```python
from build123d import *

# Parameters (mm, degrees)
F1_DEPTH = 60.325
F2_DEPTH = 11.1125
F4_DEPTH = 11.1125
F0_W     = 11.1125
F0_H     = 33.3375
F5_DEPTH = 50.8
F6_DEPTH = 25.4
F8_DEPTH = 11.1125


with BuildPart() as f1:
    # F0 (on Top) → F1 (new body)
    with BuildSketch(Plane.XY):
        Polygon((114.3, 0), (0, 0), (0, -11.1125), (11.1125, -11.1125), (63.5, -11.1125), (114.3, -11.1125), align=None)
    extrude(amount=F1_DEPTH)

    # F0 (on Top) → F2 (join)
    with BuildSketch(Plane.XY):
        Polygon((63.5, -11.1125), (11.1125, -11.1125), (11.1125, -44.45), align=None)
    extrude(amount=F2_DEPTH)

    # F3 (on face) → F4 (cut)
    with BuildSketch(Plane.XZ.offset(11.1125)):
        Polygon((114.3, 60.325), (31.75, 60.325), (114.3, 38.205794), align=None)
    extrude(amount=-F4_DEPTH, mode=Mode.SUBTRACT)

    # F0 (on Top) → F5 (join)
    with BuildSketch(Plane.XY):
        with Locations((5.55625, -27.78125)):
            Rectangle(F0_W, F0_H)
    extrude(amount=F5_DEPTH)

    # F3 (on face) → F6 (cut)
    with BuildSketch(Plane.XZ.offset(11.1125)):
        with BuildLine():
            ThreePointArc((103.1875, 19.05), (89.63734, 24.66266), (95.25, 11.1125))
            ThreePointArc((95.25, 11.1125), (100.86266, 13.43734), (103.1875, 19.05))
        make_face()
    extrude(amount=-F6_DEPTH, mode=Mode.SUBTRACT)

    # F7 (on face) → F8 (cut)
    with BuildSketch(Plane.YZ.offset(11.1125)):
        Polygon((-44.45, 50.8), (-44.45, 22.225), (-27.952216, 50.8), align=None)
    extrude(amount=-F8_DEPTH, mode=Mode.SUBTRACT)


solid = f1.part
```
Could you check a few things on this model? Use its own coordinates, in mm. A direction names the side the tool comes from. Give positions to 0.01 mm unless a question says otherwise; leave off trailing zeros. Write each loop counter-clockwise with the first axis right and the second up, starting at its lowest first coordinate (ties: lowest second). Pieces come first, ordered by that corner, then holes. Notation, with made-up numbers: (-24.75, 68.5) - (31.25, 68.5) arc R29 ccw to (31.25, 101.5) - close; hole circle Ø9 at (-39.5, 29). An arc over 180 degrees is marked (long way). One line per item, written item: value. Start each with the question number.
Item 1: Which directions (+Z, -Z, +X, -X, +Y, -Y) give clear straight access to the entire face, cutting with the end or side of a thin tool? Please do faces 1 (the face through (0, -18, 23)), 2 (the face through (11.112, -24, 31)), 3 (the face through (5, -19, 50.8)).
Item 2: Imagine slicing it at C-C, the plane z = 8. List the corners of the cut face in (x, y) for me.
Item 3: Imagine slicing it at D-D, the plane y = -19.5. List the corners of the cut face in (x, z) for me.
Item 4: Please list where these lines run through material, in increasing order: line 1 (X direction, y = -7.75, z = 19.05); line 2 (X direction, y = -22, z = 34.5). Write a range as from..to.
Item 5: I'm going to push flat-ended pins straight in: pin 1 (8 mm diameter, centred on x = 63, y = -8.5, fed in from +Z); pin 2 (10 mm diameter, centred on x = 41, z = 43, fed in from -Y); pin 3 (10 mm diameter, centred on y = -26, z = 34.5, fed in from +X); pin 4 (14.5 mm diameter, centred on x = 95.25, z = 19.05, fed in from +Y). Where does each tip first touch, or does it pass through?
Geometry says:
1. face 1: +Z, -Z, -X, +Y, -Y
1. face 2: +Z, +X, -Y
1. face 3: +Z, +X, -X, -Y
2. outline: (0, -44.45) - (11.11, -44.45) - (63.5, -11.11) - (114.3, -11.11) - (114.3, 0) - (0, 0) - close
3. outline: (0, 0) - (50.32, 0) - (50.32, 11.11) - (11.11, 11.11) - (11.11, 50.8) - (0, 50.8) - close
4. line 1: 0..87.31, 103.19..114.3
4. line 2: 0..11.11
5. pin 1: z = 53.02
5. pin 2: y = -11.11
5. pin 3: x = 11.11
5. pin 4: through
